Autodesk Inventor part; units mm, degrees
ref_plane "YZ Plane" through (0, 0, 0) normal (1, 0, 0) x (0, 1, 0)
ref_plane "XZ Plane" through (0, 0, 0) normal (0, 1, 0) x (-1, 0, 0)
ref_plane "XY Plane" through (0, 0, 0) normal (0, 0, 1) x (1, 0, 0)
sketch "스케치3" plane through (0, 0, 0) normal (0, 1, 0) x (-1, 0, 0)
  line L0 (35.5919, -14.7426) -> (14.7426, -35.5919)
  line L1 (14.7426, -35.5919) -> (-14.7426, -35.5919)
  line L2 (-14.7426, -35.5919) -> (-35.5919, -14.7426)
  line L3 (-35.5919, -14.7426) -> (-35.5919, 14.7426)
  line L4 (-35.5919, 14.7426) -> (-14.7426, 35.5919)
  line L5 (-14.7426, 35.5919) -> (14.7426, 35.5919)
  line L6 (14.7426, 35.5919) -> (35.5919, 14.7426)
  line L7 (35.5919, 14.7426) -> (35.5919, -14.7426)
  line L8 (13.5, -32.5919) -> (-13.5, -32.5919)
  line L9 (-13.5, -32.5919) -> (-32.5919, -13.5)
  line L10 (-32.5919, -13.5) -> (-32.5919, 13.5)
  line L11 (-32.5919, 13.5) -> (-13.5, 32.5919)
  line L12 (-13.5, 32.5919) -> (13.5, 32.5919)
  line L13 (13.5, 32.5919) -> (32.5919, 13.5)
  line L14 (32.5919, 13.5) -> (32.5919, -13.5)
  line L15 (32.5919, -13.5) -> (13.5, -32.5919)
  point P0 (0, 0)
  point P1 (0, 0)
  point P2 (0, 0)
  point P3 (0, 0)
  dimension "d66" = 27
  dimension "d67" = 3
extrude "돌출2" add sketch "스케치3" along normal blind 4.4 contours L0 L1 L2 L3 L4 L5 L6 L7 | L8 L9 L10 L11 L12 L13 L14 L15
sketch "스케치4" plane through (0, 4.4, 0) normal (0, 1, 0) x (1, 0, 0)
  line L0 (13.5, -32.5919) -> (-13.5, -32.5919)
  line L1 (-13.5, -32.5919) -> (-32.5919, -13.5)
  line L2 (-32.5919, -13.5) -> (-32.5919, 13.5)
  line L3 (-32.5919, 13.5) -> (-13.5, 32.5919)
  line L4 (-13.5, 32.5919) -> (13.5, 32.5919)
  line L5 (13.5, 32.5919) -> (32.5919, 13.5)
  line L6 (32.5919, 13.5) -> (32.5919, -13.5)
  line L7 (32.5919, -13.5) -> (13.5, -32.5919)
  line L8 (-14.2456, 34.3919) -> (14.2456, 34.3919)
  line L9 (14.2456, 34.3919) -> (34.3919, 14.2456)
  line L10 (34.3919, 14.2456) -> (34.3919, -14.2456)
  line L11 (34.3919, -14.2456) -> (14.2456, -34.3919)
  line L12 (14.2456, -34.3919) -> (-14.2456, -34.3919)
  line L13 (-14.2456, -34.3919) -> (-34.3919, -14.2456)
  line L14 (-34.3919, -14.2456) -> (-34.3919, 14.2456)
  line L15 (-34.3919, 14.2456) -> (-14.2456, 34.3919)
  line L16 (-13.4172, 32.3919) -> (13.4172, 32.3919)
  line L17 (13.4172, 32.3919) -> (32.3919, 13.4172)
  line L18 (32.3919, 13.4172) -> (32.3919, -13.4172)
  line L19 (32.3919, -13.4172) -> (13.4172, -32.3919)
  line L20 (13.4172, -32.3919) -> (-13.4172, -32.3919)
  line L21 (-13.4172, -32.3919) -> (-32.3919, -13.4172)
  line L22 (-32.3919, -13.4172) -> (-32.3919, 13.4172)
  line L23 (-32.3919, 13.4172) -> (-13.4172, 32.3919)
  point P0 (0, 0)
  point P1 (0, 0)
  point P2 (0, 0)
  point P3 (0, 0)
  dimension "d7" = 27
  dimension "d68" = 1.8
  dimension "d69" = 0.2
extrude "돌출3" cut sketch "스케치4" against normal blind 1.2 contours L0 L1 L2 L3 L4 L5 L6 L7 | L8 L9 L10 L11 L12 L13 L14 L15 | L16 L17 L18 L19 L20 L21 L22 L23
sketch "스케치9" plane through (0, 0, 0) normal (0, -1, 0) x (1, 0, 0)
  line L0 (7.5, 10) -> (2.5, 10)
  line L1 (2.5, 10) -> (2.5, -10)
  line L2 (2.5, -10) -> (7.5, -10)
  line L3 (7.5, -10) -> (7.5, 10)
  line L4 (7.5, 10) -> (2.5, -10) construction
  line L5 (2.5, 10) -> (7.5, -10) construction
  line L6 (-2.5, 10) -> (-7.5, 10)
  line L7 (-7.5, 10) -> (-7.5, -10)
  line L8 (-7.5, -10) -> (-2.5, -10)
  line L9 (-2.5, 10) -> (-7.5, -10) construction
  line L10 (-7.5, 10) -> (-2.5, -10) construction
  line L11 (-2.5, -10) -> (-2.5, 10)
  point P0 (0, 0)
  point P1 (5, 0)
  point P2 (-5, 0)
  dimension "d42" = 20
  dimension "d43" = 5
  dimension "d44" = 2.5
  dimension "d47" = 10
extrude "돌출8" add sketch "스케치9" along normal blind 10
sketch "스케치10" plane through (-7.5, 0, -10) normal (-1, 0, 0) x (0, 0, 1)
  circle A0 centre (15, -5) radius 1.25
  line L0 (19.9591, 0) -> (0.0886, 0)
  line L1 (24.7426, 0) -> (-4.7426, 0)
  circle A1 centre (5, -5) radius 1.25
  line L2 (20, 0) -> (20, -10)
  point P0 (10, 0)
  dimension "d54" = 2.5
  dimension "d57" = 10
  dimension "d62" = 5
  dimension "d63" = 5
extrude "돌출9" cut sketch "스케치10" against normal blind 20
sketch "스케치11" plane through (0, 3.2, 0) normal (0, 1, 0) x (1, 0, 0)
  line L0 (-13.4172, 32.3919) -> (13.4172, 32.3919)
  line L1 (13.4172, 32.3919) -> (32.3919, 13.4172)
  line L2 (32.3919, 13.4172) -> (32.3919, -13.4172)
  line L3 (32.3919, -13.4172) -> (13.4172, -32.3919)
  line L4 (13.4172, -32.3919) -> (-13.4172, -32.3919)
  line L5 (-13.4172, -32.3919) -> (-32.3919, -13.4172)
  line L6 (-32.3919, -13.4172) -> (-32.3919, 13.4172)
  line L7 (-32.3919, 13.4172) -> (-13.4172, 32.3919)
  line L8 (-14.2456, 34.3919) -> (14.2456, 34.3919)
  line L9 (-12.1745, 29.3919) -> (12.1745, 29.3919)
  line L10 (12.1745, 29.3919) -> (29.3919, 12.1745)
  line L11 (29.3919, 12.1745) -> (29.3919, -12.1745)
  line L12 (29.3919, -12.1745) -> (12.1745, -29.3919)
  line L13 (12.1745, -29.3919) -> (-12.1745, -29.3919)
  line L14 (-12.1745, -29.3919) -> (-29.3919, -12.1745)
  line L15 (-29.3919, -12.1745) -> (-29.3919, 12.1745)
  line L16 (-29.3919, 12.1745) -> (-12.1745, 29.3919)
  point P0 (0, 0)
  point P1 (0, 0)
  point P2 (0, 0)
  dimension "d70" = 2
  dimension "d71" = 3
extrude "돌출10" add sketch "스케치11" along normal blind 0.6 contours L0 L1 L2 L3 L4 L5 L6 L7 | L9 L10 L11 L12 L13 L14 L15 L16
fillet "모깎기1" radius 1.2 16 edges at (-25.1673, 4.4, 25.1673) (0, 4.4, 35.5919) (25.1673, 4.4, 25.1673) (35.5919, 4.4, 0) (25.1673, 4.4, -25.1673) (0, 4.4, -35.5919) (-25.1673, 4.4, -25.1673) (-35.5919, 4.4, 0) (-25.1673, 0, 25.1673) (0, 0, 35.5919) (25.1673, 0, 25.1673) (35.5919, 0, 0) (25.1673, 0, -25.1673) (0, 0, -35.5919) (-25.1673, 0, -25.1673) (-35.5919, 0, 0)
properties part number "OV-PAM_bottom_2"
Verification items for the finished model (mm, model axes). A direction names the side the tool comes from. Give positions to 0.01 mm unless a question says otherwise; leave off trailing zeros. Order: outer loops, then holes, each group sorted by start corner. A loop starts at its lowest first (then second) coordinate and runs counter-clockwise, first axis right, second up. Notation, with made-up numbers: M 56.25,76 L 98.25,76 A6 ccw 98.25,81 Z; hole C 40,-17.75 d11. An arc over 180 degrees is marked long. Use one line per item in the form item = value. Start each with the question number.
Q1. Access from +Z, -Z, +X, -X, +Y, -Y to the whole of each face (thin tool, end or side, straight path). Record for faces 4 (the flat face through (-5, -5, 10)), 5 (the flat face through (-7.5, -5, 0)), 6 (the flat face through (-24.46, 3.81, -24.18)).
Q2. Mould release check, pull along X, two halves, no side actions. Record for faces 1 (the flat face through (24.46, 3.81, 24.18)), 2 (the flat face through (-5, -5, -10)), 3 (the flat face through (25.313, 2.186, 25.021)): +X half, -X half, draft (parallel to the pull), parting line (faces both ways), or undercut.
Q3. Section check B-B (z = -5). Count the separate pieces of the cut face and the enclosed holes in it, then the cut area to 3 significant figures.
Q4. Go/stop test with flat-tipped pins: pin 1 Ø5 at (y, z) = (-7.5, -3) entering from +X; pin 2 Ø19.5 at (x, z) = (-7.5, -14.5) entering from +Y; pin 3 Ø0.7 at (y, z) = (3.5, 5) entering from +X; pin 4 Ø1 at (x, y) = (-19, 2.5) entering from -Z. Record where each tip stops, or that it passes through.
Q5. Section check A-A (y = -8.5). Enter the section's corners in (x, z), then the cut area to 3 significant figures.
Q6. Scan lines: line 1 along X through (y, z) = (3.25, -8); line 2 along Y through (x, z) = (-3.7, 5); line 3 along X through (y, z) = (-4, -3). Record each from-to range of solid material in increasing order. Write a range as [from, to].
Evaluation:
q1.face_4 = +Z, +X, -X, -Y
q1.face_5 = +Z, -Z, -X, -Y
q1.face_6 = +Y
q2.face_1 = undercut
q2.face_2 = draft
q2.face_3 = +X half
q3.separate_pieces = 3
q3.enclosed_holes = 0
q3.area = 343 mm2
q4.pin_1 = 7.5
q4.pin_2 = 3.8
q4.pin_3 = 35.59
q4.pin_4 = -31.83
q5.outline = M -7.5,-10 L -2.5,-10 L -2.5,10 L -7.5,10 Z; M 2.5,-10 L 7.5,-10 L 7.5,10 L 2.5,10 Z
q5.area = 200 mm2
q6.line_1 = [-35.59, -34.39], [-32.39, 32.39], [34.39, 35.59]
q6.line_2 = [-10, -6.25], [-3.75, 3.8]
q6.line_3 = [-7.5, -2.5], [2.5, 7.5]
